The listing builds one solid part. Answer for the finished solid, in the listing's coordinates (mm). A direction names the side the tool comes from. Round coordinates to 2 decimals unless told otherwise and drop trailing zeros. Order: outer loops, then holes, each group sorted by start corner. A loop starts at its lowest first (then second) coordinate and runs counter-clockwise, first axis right, second up. Notation, with made-up numbers: (-18, -35.5) - (20, -35.5) arc R17 ccw to (20, -11.5) - close; hole circle Ø4 at (-2, -24.75). An arc over 180 degrees is marked (long way). Use CSV: the item, a comma, the result in double quotes. Start each with the question number.
Item 1: Find section A-A, the plane z = 46. Give the vertices of the cut face in (x, y), plus the area to 3 significant figures.
Item 2: Find section B-B, the plane x = -33. Give the vertices of the cut face in (y, z), plus the area to 3 significant figures.
Item 3: Flat-ended cylindrical pins translate along their axes: P1, Ø3, axis at y = -5.5, z = 62.5, coming from the -X side; P2, Ø5, axis at x = 40, y = -5.5, coming from the +Z side; P3, Ø5, axis at y = -4, z = -0.5, coming from the +X side. Find the tip coordinate at first contact, or state that the pin passes through.
Item 4: Find section C-C, the plane y = -3. Give the vertices of the cut face in (x, z), plus the area to 3 significant figures.
Item 5: Straight lines are drawn through the part: line 1 along X through (y, z) = (-4, -43.5); line 2 along Z through (x, y) = (-36, -9.5); line 3 along Z through (x, y) = (-29, -8). For each, find the intervals that lie inside material, in ascending order. Write a range as [from, to].
Item 6: Find section D-D, the plane z = 17.5. Give the vertices of the cut face in (x, y).
Item 7: For faces 1 (the flat face through (30, -5, 17)), 2 (the flat face through (37, -5, -55)), 3 (the flat face through (-30, -5, -17)), 4 (the flat face through (-37, -5, 55)), 5 (the flat face through (25, -5, -45)), determine the directions among +Z, -Z, +X, -X, +Y, -Y from which every point of the face is accessible in a straight line to the end or side of a thin tool.
```python
from build123d import *

# Parameters (mm, degrees)
F0_W     = 15
F0_H     = 10
F1_DEPTH = 10


with BuildPart() as f1:
    # F0 (on Front) → F1 (new body)
    with BuildSketch(Plane.XZ):
        Polygon((30, 70), (-30, 70), (-30, 55), (-45, 55), (-45, 35), (-30, 35), (-30, -70), (30, -70), (30, -55), (45, -55), (45, -35), (30, -35), align=None)
        with Locations((32.5, -45)):
            Rectangle(F0_W, F0_H, mode=Mode.SUBTRACT)
        with Locations((-32.5, 45)):
            Rectangle(F0_W, F0_H, mode=Mode.SUBTRACT)
        Rectangle(F0_W, F0_H, mode=Mode.SUBTRACT)
    extrude(amount=F1_DEPTH)


solid = f1.part
```
Worked out:
1,outline,"(-45, -10) - (-40, -10) - (-40, 0) - (-45, 0) - close; (-25, -10) - (30, -10) - (30, 0) - (-25, 0) - close"
1,area,"600 mm²"
2,outline,"(-10, 35) - (0, 35) - (0, 40) - (-10, 40) - close; (-10, 50) - (0, 50) - (0, 55) - (-10, 55) - close"
2,area,"100 mm²"
3,P1,"stops at x = -30"
3,P2,"stops at z = -35"
3,P3,"stops at x = 30"
4,outline,"(-45, 35) - (-30, 35) - (-30, -70) - (30, -70) - (30, -55) - (45, -55) - (45, -35) - (30, -35) - (30, 70) - (-30, 70) - (-30, 55) - (-45, 55) - close; hole (-40, 40) - (-25, 40) - (-25, 50) - (-40, 50) - close; hole (-7.5, -5) - (7.5, -5) - (7.5, 5) - (-7.5, 5) - close; hole (25, -50) - (40, -50) - (40, -40) - (25, -40) - close"
4,area,"8,550 mm²"
5,line 1,"x = [-30, 25], [40, 45]"
5,line 2,"z = [35, 40], [50, 55]"
5,line 3,"z = [-70, 40], [50, 70]"
6,outline,"(-30, -10) - (30, -10) - (30, 0) - (-30, 0) - close"
7,face 1,"+Z, +X, +Y, -Y"
7,face 2,"-Z, +X, +Y, -Y"
7,face 3,"-Z, -X, +Y, -Y"
7,face 4,"+Z, -X, +Y, -Y"
7,face 5,"+Y, -Y"
